Build history of the part. All positions in model axes, mm. Face numbers are marked on the shaded views. Round coordinates to 2 decimals unless told otherwise and drop trailing zeros. Order: outer loops, then holes, each group sorted by start corner. A loop starts at its lowest first (then second) coordinate and runs counter-clockwise, first axis right, second up. Notation, with made-up numbers: (83.25, -36) -> (93.25, -36) arc R32 cw to (93.25, -5) -> close; hole circle Ø2 at (72, 72). An arc over 180 degrees is marked (long way). Use a Markdown table: item, result. Add a question column.
Item 1: Slice it at D-D, the plane y = -1.2. Give the cut face in (x, z), plus the area to 3 significant figures.
Item 2: Slice it at B-B, the plane z = -15.5. Give the cut face in (x, y), plus the area to 4 significant figures.
Item 3: Pin check, flat tips, straight feed: pin 1 (1.8 mm diameter, centred on x = -15.5, z = 15.5, fed in from -Y); pin 2 (2 mm diameter, centred on x = 8, y = -1, fed in from +Z). Stop position of each tip, or through.
Item 4: Slice it at A-A, the plane x = 0. Give the cut face in (y, z), plus the area to 3 significant figures.
Item 5: Slice it at C-C, the plane x = 15.5. Give the cut face in (y, z).
Item 6: Two-plate mould, pull along X, no slides. Class the marked faces 1 and 2: released by +X, released by -X, zero draft, split by the parting line, or undercut.
Item 7: Probe L1, parallel to X at y = 0.6, z = 15.5; L2, parallel to X at y = -0.85, z = 0; L3, parallel to X at y = -1.3, z = -15. List the from-to ranges inside material, lowest first.
from build123d import *

# Parameters (mm, degrees)
SKETCH1_R           = 12.5
SKETCH1_R_2         = 1.5
BOSS_EXTRUDE1_DEPTH = 2.5


with BuildPart() as part:
    # Sketch1 → Boss-Extrude1 (new, symmetric)
    with BuildSketch(Plane(origin=(0, 0, 0), x_dir=(1, 0, 0), z_dir=(0, 1, 0))):
        Polygon((-21.15, -21.15), (-21.15, -27.5), (-11.15, -27.5), (-11.15, -21.15), (11.15, -21.15), (11.15, -27.5), (21.15, -27.5), (21.15, -21.15), (21.15, 21.15), (-21.15, 21.15), align=None)
        with Locations(Location((0, 0, 0), (0, 0, 270))):
            Circle(SKETCH1_R, mode=Mode.SUBTRACT)
        with Locations(Location((-15.5, 15.5, 0), (0, 0, 270))):
            Circle(SKETCH1_R_2, mode=Mode.SUBTRACT)
        with Locations(Location((15.5, 15.5, 0), (0, 0, 270))):
            Circle(SKETCH1_R_2, mode=Mode.SUBTRACT)
        with Locations(Location((15.5, -15.5, 0), (0, 0, 270))):
            Circle(SKETCH1_R_2, mode=Mode.SUBTRACT)
        with Locations(Location((-15.5, -15.5, 0), (0, 0, 270))):
            Circle(SKETCH1_R_2, mode=Mode.SUBTRACT)
    extrude(amount=BOSS_EXTRUDE1_DEPTH, both=True)


solid = part.part
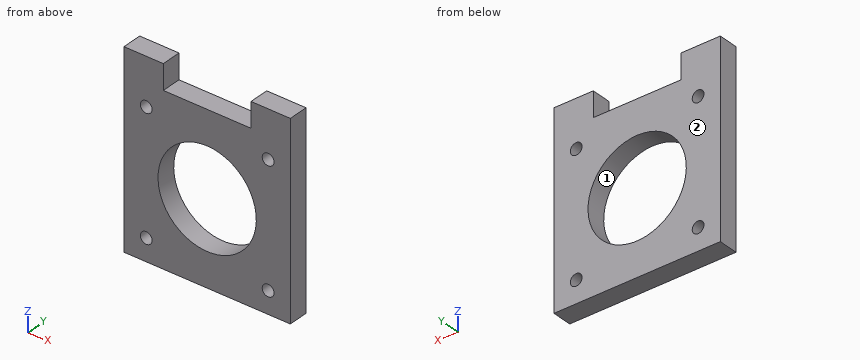
Check sheet entries:
| question | item | result |
|---|---|---|
| 1 | outline | (-21.15, -21.15) -> (21.15, -21.15) -> (21.15, 27.5) -> (11.15, 27.5) -> (11.15, 21.15) -> (-11.15, 21.15) -> (-11.15, 27.5) -> (-21.15, 27.5) -> close; hole circle Ø3 at (-15.5, -15.5); hole circle Ø3 at (-15.5, 15.5); hole circle Ø25 at (0, 0); hole circle Ø3 at (15.5, -15.5); hole circle Ø3 at (15.5, 15.5) |
| 1 | area | 1,400 mm2 |
| 2 | outline | (-21.15, -2.5) -> (-17, -2.5) -> (-17, 2.5) -> (-21.15, 2.5) -> close; (-14, -2.5) -> (14, -2.5) -> (14, 2.5) -> (-14, 2.5) -> close; (17, -2.5) -> (21.15, -2.5) -> (21.15, 2.5) -> (17, 2.5) -> close |
| 2 | area | 181.5 mm2 |
| 3 | pin 1 | through |
| 3 | pin 2 | z = 21.15 |
| 4 | outline | (-2.5, -21.15) -> (2.5, -21.15) -> (2.5, -12.5) -> (-2.5, -12.5) -> close; (-2.5, 12.5) -> (2.5, 12.5) -> (2.5, 21.15) -> (-2.5, 21.15) -> close |
| 4 | area | 86.5 mm2 |
| 5 | outline | (-2.5, -21.15) -> (2.5, -21.15) -> (2.5, -17) -> (-2.5, -17) -> close; (-2.5, -14) -> (2.5, -14) -> (2.5, 14) -> (-2.5, 14) -> close; (-2.5, 17) -> (2.5, 17) -> (2.5, 27.5) -> (-2.5, 27.5) -> close |
| 6 | face 1 | undercut |
| 6 | face 2 | zero draft |
| 7 | L1 | -21.15 to -17, -14 to 14, 17 to 21.15 |
| 7 | L2 | -21.15 to -12.5, 12.5 to 21.15 |
| 7 | L3 | -21.15 to -16.91, -14.09 to 14.09, 16.91 to 21.15 |
